```python
from build123d import *
from build123d.topology import SkipClean

# Parameters (mm, degrees)
SKETCH_1_R                      = 10
SKETCH_1_R_2                    = 2.75
EXTRUDE_1_DEPTH                 = 1.5
SKETCH_2_R                      = 10
SKETCH_2_R_2                    = 8.5
EXTRUDE_2_DEPTH                 = 3
SKETCH_3_R                      = 4.25
SKETCH_3_R_2                    = 2.75
EXTRUDE_3_DEPTH                 = 40.5
EXTRUDE_START                   = -1.5
SKETCH_4_R                      = 20
SKETCH_4_R_2                    = 8.5
SKETCH_4_R_3                    = 2
SKETCH_4_R_4                    = 1.9999999999999996
SKETCH_4_R_5                    = 2.0000000000000013
EXTRUDE_4_DEPTH                 = 1.5
EXTRUDE_START_2                 = 8
SKETCH_5_R                      = 20
SKETCH_5_R_2                    = 18.5
EXTRUDE_5_DEPTH                 = 8
EXTRUDE_START_3                 = 1.5
SKETCH_8_R                      = 41
SKETCH_8_R_2                    = 18.5
SKETCH_8_R_3                    = 0.9000000000000004
SKETCH_8_R_4                    = 0.9000000000000011
EXTRUDE_6_DEPTH                 = 1.5
SKETCH_9_R                      = 30.000000000000004
SKETCH_9_R_2                    = 29
EXTRUDE_7_DEPTH                 = 9
EXTRUDE_START_4                 = -1
SKETCH_10_R                     = 39
SKETCH_10_R_2                   = 29
EXTRUDE_8_DEPTH                 = 1
SKETCH_12_R                     = 39
SKETCH_12_R_2                   = 37.8
EXTRUDE_9_DEPTH                 = 3
EXTRUDE_START_5                 = -9
EXTRUDE_10_DEPTH                = 9
CUT_EXTRUDE_1_REACH             = 73.596
SKETCH_14_R                     = 1.0999999999999972
CUT_EXTRUDE_1_DIRECTION_2_REACH = 73.596


with BuildPart() as part:
    # 草图1 → 凸台-拉伸1 (new body)
    with BuildSketch(Plane(origin=(0, 0, 0), x_dir=(1, 0, 0), z_dir=(0, 1, 0))):
        with Locations(Location((0, 0, 0), (0, 0, 270))):
            Circle(SKETCH_1_R)
        with Locations(Location((0, 0, 0), (0, 0, 270))):
            Circle(SKETCH_1_R_2, mode=Mode.SUBTRACT)
    extrude(amount=EXTRUDE_1_DEPTH)

    # 草图2 → 凸台-拉伸2 (add)
    with BuildSketch(Plane(origin=(0, 1.5, 0), x_dir=(1, 0, 0), z_dir=(0, 1, 0))):
        with Locations(Location((0, 0, 0), (0, 0, 270))):
            Circle(SKETCH_2_R)
        with Locations(Location((0, 0, 0), (0, 0, 270))):
            Circle(SKETCH_2_R_2, mode=Mode.SUBTRACT)
    extrude(amount=EXTRUDE_2_DEPTH)

    # 草图3 → 凸台-拉伸3 (add)
    with BuildSketch(Plane(origin=(0, 1.5, 0), x_dir=(1, 0, 0), z_dir=(0, 1, 0))):
        with Locations(Location((0, 0, 0), (0, 0, 270))):
            Circle(SKETCH_3_R)
        with Locations(Location((0, 0, 0), (0, 0, 270))):
            Circle(SKETCH_3_R_2, mode=Mode.SUBTRACT)
    extrude(amount=EXTRUDE_3_DEPTH)

    # 草图4 → 凸台-拉伸4 (add)
    with BuildSketch(Plane(origin=(0, 4.500000000000001, 0), x_dir=(1, 0, 0), z_dir=(0, 1, 0)).offset(EXTRUDE_START)):
        with Locations(Location((0, 0, 0), (0, 0, 270))):
            Circle(SKETCH_4_R)
        with Locations(Location((0, 0, 0), (0, 0, 270))):
            Circle(SKETCH_4_R_2, mode=Mode.SUBTRACT)
        with Locations(Location((0, -14, 0), (0, 0, 270))):
            Circle(SKETCH_4_R_3, mode=Mode.SUBTRACT)
        with Locations(Location((-14, 0, 0), (0, 0, 270))):
            Circle(SKETCH_4_R_4, mode=Mode.SUBTRACT)
        with Locations(Location((14, 0, 0), (0, 0, 270))):
            Circle(SKETCH_4_R_5, mode=Mode.SUBTRACT)
        with Locations(Location((0, 14, 0), (0, 0, 270))):
            Circle(SKETCH_4_R_3, mode=Mode.SUBTRACT)
    extrude(amount=EXTRUDE_4_DEPTH)

    # 草图5 → 凸台-拉伸5 (add)
    with BuildSketch(Plane.XZ.offset(-3.0000000000000004).offset(EXTRUDE_START_2)):
        with Locations(Location((0, 0, 0), (0, 0, 90))):
            Circle(SKETCH_5_R)
        with Locations(Location((0, 0, 0), (0, 0, 270))):
            Circle(SKETCH_5_R_2, mode=Mode.SUBTRACT)
    extrude(amount=-EXTRUDE_5_DEPTH)

    # 草图8 → 凸台-拉伸6 (add)
    with BuildSketch(Plane.XZ.offset(4.999999999999999).offset(EXTRUDE_START_3)):
        with Locations(Location((0, 0, 0), (0, 0, 270))):
            Circle(SKETCH_8_R)
        with Locations(Location((0, 0, 0), (0, 0, 270))):
            Circle(SKETCH_8_R_2, mode=Mode.SUBTRACT)
        with Locations(Location((24, 0, 0), (0, 0, 270))):
            Circle(SKETCH_8_R_3, mode=Mode.SUBTRACT)
        with Locations(Location((-24, 0, 0), (0, 0, 270))):
            Circle(SKETCH_8_R_3, mode=Mode.SUBTRACT)
        with Locations(Location((0, -24, 0), (0, 0, 270))):
            Circle(SKETCH_8_R_4, mode=Mode.SUBTRACT)
        with Locations(Location((0, 24, 0), (0, 0, 270))):
            Circle(SKETCH_8_R_4, mode=Mode.SUBTRACT)
        Polygon((9.192388155425043, -21.92031021678299), (21.92031021678307, -9.192388155425377), (25.455844122715792, -12.727922061358134), (12.727922061357729, -25.455844122715785), align=None, mode=Mode.SUBTRACT)
    extrude(amount=-EXTRUDE_6_DEPTH)

    # 草图9 → 凸台-拉伸7 (add)
    with BuildSketch(Plane(origin=(0, -4.999999999999999, 0), x_dir=(1, 0, 0), z_dir=(0, 1, 0))):
        with Locations(Location((0, 0, 0), (0, 0, 90))):
            Circle(SKETCH_9_R)
        with Locations(Location((0, 0, 0), (0, 0, 270))):
            Circle(SKETCH_9_R_2, mode=Mode.SUBTRACT)
    extrude(amount=EXTRUDE_7_DEPTH)

    # 草图10 → 凸台-拉伸8 (add)
    with BuildSketch(Plane(origin=(0, 4, 0), x_dir=(1, 0, 0), z_dir=(0, 1, 0)).offset(EXTRUDE_START_4)):
        with Locations(Location((0, 0, 0), (0, 0, 270))):
            Circle(SKETCH_10_R)
        with Locations(Location((0, 0, 0), (0, 0, 270))):
            Circle(SKETCH_10_R_2, mode=Mode.SUBTRACT)
    extrude(amount=EXTRUDE_8_DEPTH)

    # 草图12 → 凸台-拉伸9 (add)
    with BuildSketch(Plane(origin=(0, -4.999999999999999, 0), x_dir=(1, 0, 0), z_dir=(0, 1, 0))):
        with Locations(Location((0, 0, 0), (0, 0, 270))):
            Circle(SKETCH_12_R)
        with Locations(Location((0, 0, 0), (0, 0, 270))):
            Circle(SKETCH_12_R_2, mode=Mode.SUBTRACT)
    extrude(amount=EXTRUDE_9_DEPTH)

    # 草图13 → 凸台-拉伸10 (add)
    with SkipClean():  # the faces are left unmerged after this step: merging them gives an invalid solid
        with BuildSketch(Plane(origin=(0, 4, 0), x_dir=(1, 0, 0), z_dir=(0, 1, 0)).offset(EXTRUDE_START_5)):
            with BuildLine():
                Line((1.923076923076923, 37.45065787336625), (2, 38.948684188300895))
                ThreePointArc((2, 38.948684188300895), (2.39e-15, 39), (-2, 38.948684188300895))
                Line((-2, 38.948684188300895), (-1.923076923076923, 37.45065787336625))
                ThreePointArc((-1.923076923076923, 37.45065787336625), (2.3e-15, 37.5), (1.923076923076923, 37.45065787336625))
            make_face()
            with BuildLine():
                Line((25.12179340910359, 27.8414348752057), (26.12666514546773, 28.955092270213918))
                ThreePointArc((26.12666514546773, 28.955092270213918), (27.577164466275356, 27.577164466275352), (28.955092270213918, 26.12666514546773))
                Line((28.955092270213918, 26.12666514546773), (27.841434875205692, 25.12179340910359))
                ThreePointArc((27.841434875205692, 25.12179340910359), (26.516504294495533, 26.51650429449554), (25.12179340910359, 27.8414348752057))
            make_face()
            with BuildLine():
                Line((37.45065787336625, 1.9230769230769253), (38.948684188300895, 2.0000000000000027))
                ThreePointArc((38.948684188300895, 2.0000000000000027), (39, 2.71e-15), (38.948684188300895, -1.9999999999999973))
                Line((38.948684188300895, -1.9999999999999973), (37.45065787336625, -1.923076923076921))
                ThreePointArc((37.45065787336625, -1.923076923076921), (37.5, 2.08e-15), (37.45065787336625, 1.9230769230769253))
            make_face()
            with BuildLine():
                Line((27.8414348752057, -25.12179340910359), (28.955092270213918, -26.126665145467726))
                ThreePointArc((28.955092270213918, -26.126665145467726), (27.577164466275356, -27.577164466275352), (26.12666514546773, -28.955092270213914))
                Line((26.12666514546773, -28.955092270213914), (25.12179340910359, -27.841434875205692))
                ThreePointArc((25.12179340910359, -27.841434875205692), (26.51650429449554, -26.516504294495533), (27.8414348752057, -25.12179340910359))
            make_face()
            with BuildLine():
                Line((1.9230769230769276, -37.45065787336625), (2.0000000000000044, -38.948684188300895))
                ThreePointArc((2.0000000000000044, -38.948684188300895), (2.39e-15, -39), (-1.9999999999999958, -38.948684188300895))
                Line((-1.9999999999999958, -38.948684188300895), (-1.9230769230769182, -37.45065787336625))
                ThreePointArc((-1.9230769230769182, -37.45065787336625), (2.3e-15, -37.5), (1.9230769230769276, -37.45065787336625))
            make_face()
            with BuildLine():
                Line((-25.12179340910359, -27.841434875205703), (-26.126665145467726, -28.95509227021392))
                ThreePointArc((-26.126665145467726, -28.95509227021392), (-27.577164466275352, -27.577164466275356), (-28.955092270213914, -26.126665145467733))
                Line((-28.955092270213914, -26.126665145467733), (-27.841434875205692, -25.121793409103592))
                ThreePointArc((-27.841434875205692, -25.121793409103592), (-26.516504294495533, -26.51650429449554), (-25.12179340910359, -27.841434875205703))
            make_face()
            with BuildLine():
                Line((-37.45065787336625, -1.9230769230769298), (-38.948684188300895, -2.000000000000007))
                ThreePointArc((-38.948684188300895, -2.000000000000007), (-39, -1.254e-14), (-38.948684188300895, 1.9999999999999931))
                Line((-38.948684188300895, 1.9999999999999931), (-37.45065787336625, 1.923076923076916))
                ThreePointArc((-37.45065787336625, 1.923076923076916), (-37.5, -1.206e-14), (-37.45065787336625, -1.9230769230769298))
            make_face()
            with BuildLine():
                Line((-27.841434875205703, 25.12179340910358), (-28.95509227021392, 26.126665145467722))
                ThreePointArc((-28.95509227021392, 26.126665145467722), (-27.577164466275352, 27.577164466275356), (-26.126665145467733, 28.95509227021391))
                Line((-26.126665145467733, 28.95509227021391), (-25.121793409103592, 27.84143487520569))
                ThreePointArc((-25.121793409103592, 27.84143487520569), (-26.516504294495547, 26.516504294495526), (-27.841434875205703, 25.12179340910358))
            make_face()
        extrude(amount=EXTRUDE_10_DEPTH)

    # 草图14 → 切除-拉伸1 (cut, up to next)
    with BuildSketch(Plane(origin=(0, 0, 0), x_dir=(0, 0, -1), z_dir=(1, 0, 0)), mode=Mode.PRIVATE) as cut_extrude_1_sk1:
        with Locations((0, 39)):
            Circle(SKETCH_14_R)
    cut_extrude_1_tool1 = extrude(cut_extrude_1_sk1.sketch, amount=-CUT_EXTRUDE_1_REACH, mode=Mode.PRIVATE) & part.part
    add(cut_extrude_1_tool1.solids().sort_by_distance((0, 39, 0))[0], mode=Mode.SUBTRACT)

    # 草图14 → 切除-拉伸1 direction 2 (cut, up to next)
    with BuildSketch(Plane(origin=(0, 0, 0), x_dir=(0, 0, -1), z_dir=(1, 0, 0)), mode=Mode.PRIVATE) as cut_extrude_1_direction_2_sk1:
        with Locations((0, 39)):
            Circle(SKETCH_14_R)
    cut_extrude_1_direction_2_tool1 = extrude(cut_extrude_1_direction_2_sk1.sketch, amount=CUT_EXTRUDE_1_DIRECTION_2_REACH, mode=Mode.PRIVATE) & part.part
    add(cut_extrude_1_direction_2_tool1.solids().sort_by_distance((0, 39, 0))[0], mode=Mode.SUBTRACT)


solid = part.part
```
Can you work these out from the model? Positions are in its coordinate system, mm. A direction names the side the tool comes from. Coordinates: 2 decimals unless noted, no trailing zeros. Loops run counter-clockwise (first coordinate to the right, second up) from the corner with the lowest first, then second, coordinate; pieces in that order, holes last. Notation, with made-up numbers: (-4.75, -30) - (31.25, -30) arc R12 ccw to (31.25, -15) - close; hole circle Ø1 at (-11.5, -24.75). An arc over 180 degrees is marked (long way). Use a Markdown table: item, result.
Item 1: We'd pull the mould along Z, two halves only. Please class faces 1 (the face through (-40, -6, 9)), 2 (the face through (-1.2, 3.7, 12.4)), 3 (the face through (-3, 42, 0)): released by +Z, released by -Z, zero draft, split by the parting line, or undercut.
Numbers:
| item | result |
|---|---|
| face 1 | split by the parting line |
| face 2 | undercut |
| face 3 | zero draft |
Item 2: I want a section at C-C on x = 14. Give the number of separate pieces and of enclosed holes in the cut face, and give its area (3 significant figures).
Numbers:
| item | result |
|---|---|
| separate pieces | 3 |
| enclosed holes | 0 |
| area | 189 mm2 |
Item 3: I want a section at B-B on y = 22.5. Please give me the cut outline in (x, z), and give its area (3 significant figures).
Numbers:
| item | result |
|---|---|
| outline | circle Ø8.5 at (0, 0); hole circle Ø5.5 at (0, 0) |
| area | 33.0 mm2 |
Item 4: If I drill on probe 1 along X at (y, z) = (4.05, 0); probe 2 along Y at (x, z) = (18, -27.5); probe 3 along Z at (x, y) = (17, 3.5), over which ranges is the centre line in solid material (lowest first)? Write a range as from..to.
Numbers:
| item | result |
|---|---|
| probe 1 | x = -20..-16, -12..-8.5, -4.25..-2.75, 2.75..4.25, 8.5..12, 16..20 |
| probe 2 | y = -6.5..-5, 3..4 |
| probe 3 | z = -35.1..-23.49, -10.54..10.54, 23.49..35.1 |
Item 5: Will these pins go through, and if not, where does the flat tip stop? pin 1 (19.5 mm diameter, centred on x = 0, z = 0, fed in from -Y); pin 2 (8 mm diameter, centred on x = 5.5, z = -12, fed in from +Y); pin 3 (1.2 mm diameter, centred on x = 0.5, z = -38, fed in from +Y).
Numbers:
| item | result |
|---|---|
| pin 1 | stops at y = 0 |
| pin 2 | stops at y = 4.5 |
| pin 3 | stops at y = 4 |
Item 6: I want a section at A-A on y = 39. Please give me the cut outline in (x, z), and give its area (3 significant figures).
Numbers:
| item | result |
|---|---|
| outline | (-4.11, -1.1) arc R4.25 ccw to (4.11, -1.1) - (2.52, -1.1) arc R2.75 cw to (-2.52, -1.1) - close; (-4.11, 1.1) - (-2.52, 1.1) arc R2.75 cw to (2.52, 1.1) - (4.11, 1.1) arc R4.25 ccw to start |
| area | 26.3 mm2 |
Item 7: For faces 4 (the face through (37.5, -1.1, 0)), 5 (the face through (19.181, -5.76, -19.003)), 6 (the face through (-8, 3, 8)), which set-ups out of +Z, -Z, +X, -X, +Y, -Y let a thin tool reach every point of the face, with its end or its side?
Numbers:
| item | result |
|---|---|
| face 4 | none |
| face 5 | +Y, -Y |
| face 6 | -Y |
